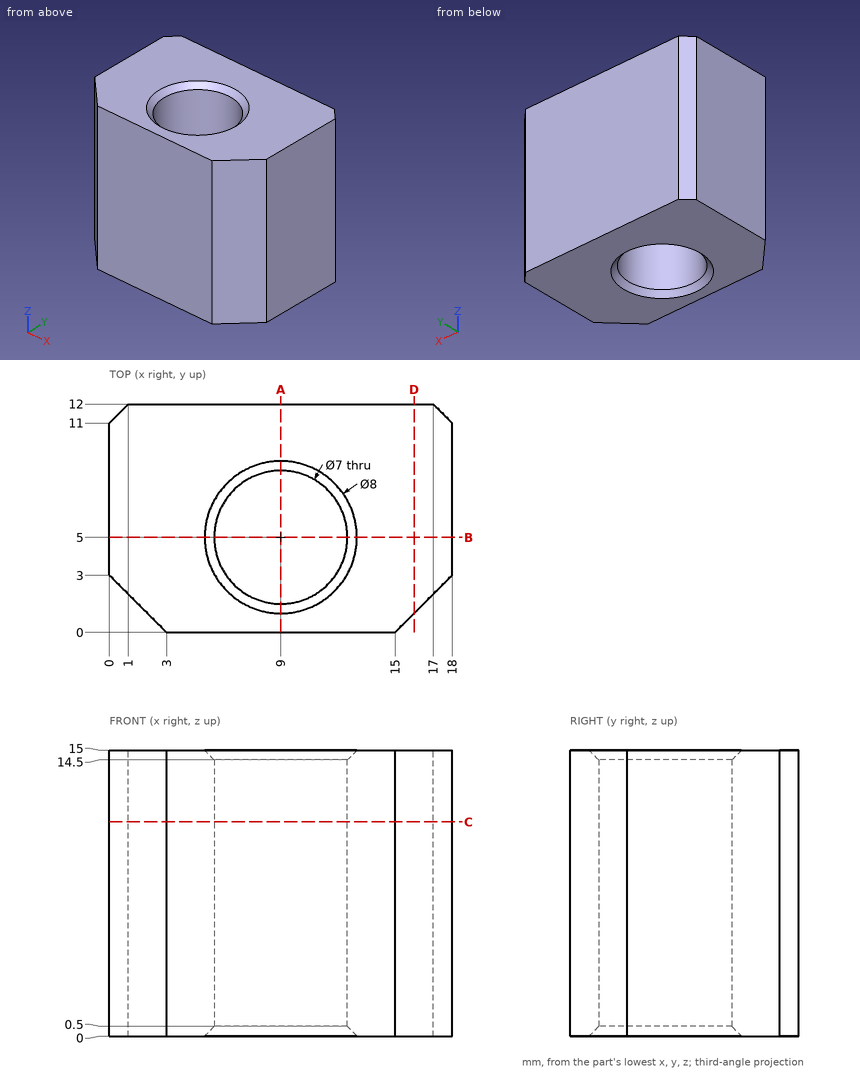
Study the drawing (mm; zero at the part's minimum x, y, z) and answer. Round coordinates to 2 decimals unless told otherwise and drop trailing zeros. Write each loop counter-clockwise with the first axis right and the second up, starting at its lowest first coordinate (ties: lowest second). Pieces come first, ordered by that corner, then holes.
Q1. Find section B-B on y = 5. Determine the outline of the cut face in (x, z).
Values:
outline: (0, 0) - (5, 0) - (5.5, 0.5) - (5.5, 14.5) - (5, 15) - (0, 15) - close; (12.5, 0.5) - (13, 0) - (18, 0) - (18, 15) - (13, 15) - (12.5, 14.5) - close
Q2. Find section A-A on x = 9. Determine the outline of the cut face in (y, z), and give its area (3 significant figures).
Values:
outline: (0, 0) - (1, 0) - (1.5, 0.5) - (1.5, 14.5) - (1, 15) - (0, 15) - close; (8.5, 0.5) - (9, 0) - (12, 0) - (12, 15) - (9, 15) - (8.5, 14.5) - close
area: 74.5 mm2
Q3. Straight lines are drawn through the part: line 1 (Y direction, x = 9, z = 4.75); line 2 (Y direction, x = 11, z = 11); line 3 (X direction, y = 2, z = 12.75). For each, find the intervals that lie inside material, in ascending order.
Values:
line 1: y = 0 to 1.5, 8.5 to 12
line 2: y = 0 to 2.13, 7.87 to 12
line 3: x = 1 to 7.2, 10.8 to 17
Q4. Find section C-C on z = 11.25. Determine the outline of the cut face in (x, y), and give its area (3 significant figures).
Values:
outline: (0, 3) - (3, 0) - (15, 0) - (18, 3) - (18, 11) - (17, 12) - (1, 12) - (0, 11) - close; hole circle Ø7 at (9, 5)
area: 168 mm2
Q5. Find section D-D on x = 16. Determine the outline of the cut face in (y, z).
Values:
outline: (1, 0) - (12, 0) - (12, 15) - (1, 15) - close
Q6. A flat-ended cylindrical pin translates along its axis: P1, Ø1.5, axis at x = 3.5, z = 11, coming from the -Y side. Find the tip coordinate at first contact, or state that the pin passes through.
Values:
P1: stops at y = 0
